from build123d import *

# Parameters (mm, degrees)
SKETCH_1_R                     = 30
EXTRUDE_1_DEPTH                = 4
EXTRUDE_2_DEPTH                = 1.9
CHAMFER_1_SIZE                 = 1
SKETCH_5_R                     = 16
CUT_EXTRUDE_2_DEPTH            = 43.83468221
HOLE_WIZARD_M2_5_1_D           = 2.7
HOLE_WIZARD_M2_5_1_CBORE_D     = 5
HOLE_WIZARD_M2_5_1_CBORE_DEPTH = 2.9
SKETCH_8_OUTSIDE_W             = 79.012
SKETCH_8_OUTSIDE_H             = 79.012
CUT_EXTRUDE_3_DEPTH            = 43.83468221
CHAMFER_2_SIZE                 = 1
SKETCH_9_R                     = 18.55
CUT_EXTRUDE_4_DEPTH            = 2.5
CHAMFER_3_SIZE                 = 0.5


with BuildPart() as part:
    # 草图1 → 凸台-拉伸1 (new body)
    with BuildSketch(Plane.YZ):
        with Locations(Location((0, 0, 0), (0, 0, 270))):
            Circle(SKETCH_1_R)
    extrude(amount=EXTRUDE_1_DEPTH)

    # 草图2 → 凸台-拉伸2 (add)
    with BuildSketch(Plane(origin=(0, 0, 0), x_dir=(0, -1, 0), z_dir=(-1, 0, 0))):
        with BuildLine():
            ThreePointArc((-15.429362873, -21.236696102), (-14.556584324, -21.641903091), (-13.595407183, -21.687439927))
            ThreePointArc((-13.595407183, -21.687439927), (-8.168716079, -21.262073185), (-2.734521388, -21.577416267))
            ThreePointArc((-2.734521388, -21.577416267), (0, -21.75), (2.734521388, -21.577416267))
            ThreePointArc((2.734521388, -21.577416267), (8.168716079, -21.262073185), (13.595407183, -21.687439927))
            ThreePointArc((13.595407183, -21.687439927), (14.556584324, -21.641903091), (15.429362873, -21.236696102))
            ThreePointArc((15.429362873, -21.236696102), (18.561553006, -18.561553006), (21.236696102, -15.429362873))
            ThreePointArc((21.236696102, -15.429362873), (21.641903091, -14.556584324), (21.687439927, -13.595407183))
            ThreePointArc((21.687439927, -13.595407183), (21.262073185, -8.168716079), (21.577416267, -2.734521388))
            ThreePointArc((21.577416267, -2.734521388), (21.75, 0), (21.577416267, 2.734521388))
            ThreePointArc((21.577416267, 2.734521388), (21.262073185, 8.168716079), (21.687439927, 13.595407183))
            ThreePointArc((21.687439927, 13.595407183), (21.641903091, 14.556584324), (21.236696102, 15.429362873))
            ThreePointArc((21.236696102, 15.429362873), (18.561553006, 18.561553006), (15.429362873, 21.236696102))
            ThreePointArc((15.429362873, 21.236696102), (14.556584324, 21.641903091), (13.595407183, 21.687439927))
            ThreePointArc((13.595407183, 21.687439927), (8.168716079, 21.262073185), (2.734521388, 21.577416267))
            ThreePointArc((2.734521388, 21.577416267), (0, 21.75), (-2.734521388, 21.577416267))
            ThreePointArc((-2.734521388, 21.577416267), (-8.168716079, 21.262073185), (-13.595407183, 21.687439927))
            ThreePointArc((-13.595407183, 21.687439927), (-14.556584324, 21.641903091), (-15.429362873, 21.236696102))
            ThreePointArc((-15.429362873, 21.236696102), (-18.561553006, 18.561553006), (-21.236696102, 15.429362873))
            ThreePointArc((-21.236696102, 15.429362873), (-21.641903091, 14.556584324), (-21.687439927, 13.595407183))
            ThreePointArc((-21.687439927, 13.595407183), (-21.262073185, 8.168716079), (-21.577416267, 2.734521388))
            ThreePointArc((-21.577416267, 2.734521388), (-21.75, 0), (-21.577416267, -2.734521388))
            ThreePointArc((-21.577416267, -2.734521388), (-21.262073185, -8.168716079), (-21.687439927, -13.595407183))
            ThreePointArc((-21.687439927, -13.595407183), (-21.641903091, -14.556584324), (-21.236696102, -15.429362873))
            ThreePointArc((-21.236696102, -15.429362873), (-18.561553006, -18.561553006), (-15.429362873, -21.236696102))
        make_face()
    extrude(amount=EXTRUDE_2_DEPTH)

    # 倒角1
    chamfer_1_edges = [part.edges().sort_by_distance(p)[0] for p in [
        (0, 21.641903091, -14.556584324),
        (0, 18.561553006, -18.561553006),
        (0, 14.556584324, -21.641903091),
        (0, 8.168716079, -21.262073185),
        (0, 0, -21.75),
        (0, -8.168716079, -21.262073185),
        (0, -14.556584324, -21.641903091),
        (0, -18.561553006, -18.561553006),
        (0, -21.641903091, -14.556584324),
        (0, -21.262073185, -8.168716079),
        (0, -21.75, 0),
        (0, -21.262073185, 8.168716079),
        (0, -21.641903091, 14.556584324),
        (0, -18.561553006, 18.561553006),
        (0, -14.556584324, 21.641903091),
        (0, -8.168716079, 21.262073185),
        (0, 0, 21.75),
        (0, 8.168716079, 21.262073185),
        (0, 14.556584324, 21.641903091),
        (0, 18.561553006, 18.561553006),
        (0, 21.641903091, 14.556584324),
        (0, 21.262073185, 8.168716079),
        (0, 21.75, 0),
        (0, 21.262073185, -8.168716079),
    ]]
    chamfer(chamfer_1_edges, length=CHAMFER_1_SIZE)

    # 草图5 → 切除-拉伸2 (cut, through all)
    with BuildSketch(Plane.YZ.offset(4)):
        with Locations(Location((0, 0, 0), (0, 0, 270))):
            Circle(SKETCH_5_R)
    extrude(amount=-CUT_EXTRUDE_2_DEPTH, mode=Mode.SUBTRACT)

    # M2.5 六角圆柱头螺钉的柱形沉头孔1 (through all)
    with Locations(Plane.YZ.offset(4)):
        with Locations((-13.959899742, 19.214153616), (13.959899742, 19.214153616), (19.214153616, 13.959899742), (19.214153616, -13.959899742), (13.959899742, -19.214153616), (-13.959899742, -19.214153616), (-19.214153616, -13.959899742), (-19.214153616, 13.959899742)):
            CounterBoreHole(HOLE_WIZARD_M2_5_1_D / 2, HOLE_WIZARD_M2_5_1_CBORE_D / 2, HOLE_WIZARD_M2_5_1_CBORE_DEPTH)

    # 草图8 outside → 切除-拉伸3 (cut, through all)
    with BuildSketch(Plane(origin=(4, 0, 0), x_dir=(0, 0, -1), z_dir=(1, 0, 0))):
        Rectangle(SKETCH_8_OUTSIDE_W, SKETCH_8_OUTSIDE_H)
        with BuildLine():
            ThreePointArc((-3.111696751, 24.553611615), (-8.138326841, 24.261919263), (-13.158016112, 24.6553835))
            ThreePointArc((-13.158016112, 24.6553835), (-15.272605822, 24.55520246), (-17.19271863, 23.663747085))
            ThreePointArc((-17.19271863, 23.663747085), (-20.68287335, 20.68287335), (-23.663747085, 17.19271863))
            ThreePointArc((-23.663747085, 17.19271863), (-24.55520246, 15.272605822), (-24.6553835, 13.158016112))
            ThreePointArc((-24.6553835, 13.158016112), (-24.261919263, 8.138326841), (-24.553611615, 3.111696751))
            ThreePointArc((-24.553611615, 3.111696751), (-24.75, 0), (-24.553611615, -3.111696751))
            ThreePointArc((-24.553611615, -3.111696751), (-24.261919263, -8.138326841), (-24.6553835, -13.158016112))
            ThreePointArc((-24.6553835, -13.158016112), (-24.55520246, -15.272605822), (-23.663747085, -17.19271863))
            ThreePointArc((-23.663747085, -17.19271863), (-20.68287335, -20.68287335), (-17.19271863, -23.663747085))
            ThreePointArc((-17.19271863, -23.663747085), (-15.272605822, -24.55520246), (-13.158016112, -24.6553835))
            ThreePointArc((-13.158016112, -24.6553835), (-8.138326841, -24.261919263), (-3.111696751, -24.553611615))
            ThreePointArc((-3.111696751, -24.553611615), (0, -24.75), (3.111696751, -24.553611615))
            ThreePointArc((3.111696751, -24.553611615), (8.138326841, -24.261919263), (13.158016112, -24.6553835))
            ThreePointArc((13.158016112, -24.6553835), (15.272605822, -24.55520246), (17.19271863, -23.663747085))
            ThreePointArc((17.19271863, -23.663747085), (20.68287335, -20.68287335), (23.663747085, -17.19271863))
            ThreePointArc((23.663747085, -17.19271863), (24.55520246, -15.272605822), (24.6553835, -13.158016112))
            ThreePointArc((24.6553835, -13.158016112), (24.261919263, -8.138326841), (24.553611615, -3.111696751))
            ThreePointArc((24.553611615, -3.111696751), (24.75, 0), (24.553611615, 3.111696751))
            ThreePointArc((24.553611615, 3.111696751), (24.261919263, 8.138326841), (24.6553835, 13.158016112))
            ThreePointArc((24.6553835, 13.158016112), (24.55520246, 15.272605822), (23.663747085, 17.19271863))
            ThreePointArc((23.663747085, 17.19271863), (20.68287335, 20.68287335), (17.19271863, 23.663747085))
            ThreePointArc((17.19271863, 23.663747085), (15.272605822, 24.55520246), (13.158016112, 24.6553835))
            ThreePointArc((13.158016112, 24.6553835), (8.138326841, 24.261919263), (3.111696751, 24.553611615))
            ThreePointArc((3.111696751, 24.553611615), (0, 24.75), (-3.111696751, 24.553611615))
        make_face(mode=Mode.SUBTRACT)
    extrude(amount=-CUT_EXTRUDE_3_DEPTH, mode=Mode.SUBTRACT)

    # 倒角2
    chamfer_2_edges = [part.edges().sort_by_distance(p)[0] for p in [
        (4, 24.75, 0),
        (4, 24.261919263, -8.138326841),
        (4, 24.55520246, -15.272605822),
        (4, 20.68287335, -20.68287335),
        (4, 15.272605822, -24.55520246),
        (4, 8.138326841, -24.261919263),
        (4, 0, -24.75),
        (4, -8.138326841, -24.261919263),
        (4, -15.272605822, -24.55520246),
        (4, -20.68287335, -20.68287335),
        (4, -24.55520246, -15.272605822),
        (4, -24.261919263, -8.138326841),
        (4, -24.75, 0),
        (4, -24.261919263, 8.138326841),
        (4, -24.55520246, 15.272605822),
        (4, -20.68287335, 20.68287335),
        (4, -15.272605822, 24.55520246),
        (4, -8.138326841, 24.261919263),
        (4, 0, 24.75),
        (4, 8.138326841, 24.261919263),
        (4, 15.272605822, 24.55520246),
        (4, 20.68287335, 20.68287335),
        (4, 24.55520246, 15.272605822),
        (4, 24.261919263, 8.138326841),
    ]]
    chamfer(chamfer_2_edges, length=CHAMFER_2_SIZE)

    # 草图9 → 切除-拉伸4 (cut)
    with BuildSketch(Plane(origin=(4, 0, 0), x_dir=(0, 0, -1), z_dir=(1, 0, 0))):
        Circle(SKETCH_9_R)
    extrude(amount=-CUT_EXTRUDE_4_DEPTH, mode=Mode.SUBTRACT)

    # 倒角3
    chamfer_3_edges = [part.edges().sort_by_distance(p)[0] for p in [
        (-1.9, 0, 16),
        (1.5, 0, 16),
    ]]
    chamfer(chamfer_3_edges, length=CHAMFER_3_SIZE)


solid = part.part
For this review, take the finished solid that the model builds, in its own axes (mm). A direction names the side the tool comes from. Give positions to 0.01 mm unless a question says otherwise; leave off trailing zeros. Order: outer loops, then holes, each group sorted by start corner. A loop starts at its lowest first (then second) coordinate and runs counter-clockwise, first axis right, second up. Notation, with made-up numbers: M 89,14.25 L 97,14.25 A7 cw 97,23.25 Z; hole C -4.5,38 d7. An arc over 180 degrees is marked long. Answer in a Markdown table with one row per item. Add a question column.
(1) For pin 1 (3 mm diameter, centred on y = 19.21, z = 13.96, fed in from -X); pin 2 (2 mm diameter, centred on x = 1.5, z = -13, fed in from +Y); pin 3 (4.5 mm diameter, centred on y = -19.21, z = -13.96, fed in from +X); pin 4 (1.5 mm diameter, centred on x = 1.5, y = -14, fed in from -Z), all flat-tipped, find the tip position at first contact; note any pin that passes through.
(2) Consider section A-A on z = 0. State the section outline as (x, y) points, and give its area (3 significant figures).
(3) For faces 4 (the face through (1.521, -24.263, 8.209)), 5 (the face through (-1.444, -18.521, -18.602)), 6 (the face through (1.1, -13, 18)), list the 3-axis set-ups (+Z, -Z, +X, -X, +Y, -Y) from which the entire face can be reached by the end or side of a thin tool; tool diameter is ignored.
(4) Wall thickness on probe 1 along Z at (x, y) = (3.5, 15.5); probe 2 along Z at (x, y) = (2.25, -16); probe 3 along X at (y, z) = (-4.5, 23): over which ranges is each line inside the solid? List them lowest first. Write a range as [from, to].
(5) Mouldability with a two-part tool opening along Y and no side actions: class faces 1 (the face through (1.521, 24.263, -8.209)), 2 (the face through (2.57, 21.6, -13.21)), 3 (the face through (-1.444, -18.602, 18.521)) as +Y half, -Y half, draft (parallel to the pull), parting line (faces both ways), or undercut.
Evaluation:
| question | item | result |
|---|---|---|
| 1 | pin 1 | stops at x = -1.9 |
| 1 | pin 2 | stops at y = 24.71 |
| 1 | pin 3 | stops at x = 1.1 |
| 1 | pin 4 | stops at z = -24.71 |
| 2 | outline | M -1.9,-21.75 L -1,-21.75 L 0,-22.75 L 0,-24.75 L 3,-24.75 L 4,-23.75 L 4,-18.55 L 1.5,-18.55 L 1.5,-16.5 L 1,-16 L -1.4,-16 L -1.9,-16.5 Z; M -1.9,16.5 L -1.4,16 L 1,16 L 1.5,16.5 L 1.5,18.55 L 4,18.55 L 4,23.75 L 3,24.75 L 0,24.75 L 0,22.75 L -1,21.75 L -1.9,21.75 Z |
| 2 | area | 78.6 mm^2 |
| 3 | face 4 | +X, -X, -Y |
| 3 | face 5 | -Z, -X, -Y |
| 3 | face 6 | +X |
| 4 | probe 1 | z = [-23.97, -21.18], [-17.24, -10.19], [10.19, 17.24], [21.18, 23.97] |
| 4 | probe 2 | z = [-24.32, -20.66], [-17.77, -9.39], [9.39, 17.77], [20.66, 24.32] |
| 4 | probe 3 | x = [0, 4] |
| 5 | face 1 | +Y half |
| 5 | face 2 | undercut |
| 5 | face 3 | -Y half |
